from build123d import *

# Parameters (mm, degrees)
SKETCH1_R           = 95.25
SKETCH1_R_2         = 76.2
BOSS_EXTRUDE1_DEPTH = 7.874
SKETCH2_R           = 3.3655
CUT_EXTRUDE1_DEPTH  = 8.874
CIRPATTERN1_COUNT   = 8


with BuildPart() as part:
    # Sketch1 → Boss-Extrude1 (new body)
    with BuildSketch(Plane.XY):
        Circle(SKETCH1_R)
        Circle(SKETCH1_R_2, mode=Mode.SUBTRACT)
    extrude(amount=BOSS_EXTRUDE1_DEPTH)

    # Sketch2 → Cut-Extrude1 (cut, through all)
    with BuildSketch(Plane.XY.offset(7.874)):
        with Locations((0, 85.09)):
            Circle(SKETCH2_R)
    cut_extrude1 = extrude(amount=-CUT_EXTRUDE1_DEPTH, mode=Mode.SUBTRACT)

    # CirPattern1: Cut-Extrude1 ×8 about axis
    cirpattern1_axis = Axis((0, 0, 0), (0, 0, 1))
    for i in range(1, CIRPATTERN1_COUNT):
        add(cut_extrude1.rotate(cirpattern1_axis, i * 360 / CIRPATTERN1_COUNT), mode=Mode.SUBTRACT)


solid = part.part
Geometry: final body of the model. Coordinates: model frame, mm. Round coordinates to 2 decimals unless told otherwise and drop trailing zeros. Loops run counter-clockwise (first coordinate to the right, second up) from the corner with the lowest first, then second, coordinate; pieces in that order, holes last. Notation, with made-up numbers: (-2.75, 51.5) - (32.25, 51.5) arc R27 ccw to (32.25, 72.5) - close; hole circle Ø8 at (20, -10.75). An arc over 180 degrees is marked (long way). Write each question's results on one line, items separated by ' | '. Start each with the question number.
1) First-contact query: P1, Ø4, axis at x = 3.5, z = 4.5, coming from the +Y side; P2, Ø7.5, axis at x = -60.17, y = 60.17, coming from the +Z side; P3, Ø4, axis at x = -85.09, y = 0, coming from the -Z side; P4, Ø2, axis at x = -31.5, z = 4.5, coming from the -Y side. Flat tips, straight axial feed; report the tip coordinate or a pass-through.
2) Cut plane A-A on y = 0. Return loops of the section in (x, z), then the cut area to 3 significant figures.
3) Line query: probe 1 along Y at (x, z) = (0, 3.5); probe 2 along Y at (x, z) = (61, 6); probe 3 along X at (y, z) = (62.5, 2). Output: solid intervals per line, ascending. Write a range as [from, to].
4) Mould query, pull axis Y, two halves, no side actions, for faces 1 (the face through (-60.47, -46.367, 3.882)), 2 (the face through (-75.587, -57.958, 3.882)), 3 (the face through (-29, 71, 0)). Classes: released by +Y, released by -Y, zero draft, split by the parting line, or undercut.
5) Cut plane C-C on y = -85.09. Return loops of the section in (x, z).
Verdict:
1) P1: stops at y = 95.24 | P2: stops at z = 7.87 | P3: passes through | P4: stops at y = -90.23
2) outline: (-95.25, 0) - (-88.46, 0) - (-88.46, 7.87) - (-95.25, 7.87) - close; (-81.72, 0) - (-76.2, 0) - (-76.2, 7.87) - (-81.72, 7.87) - close; (76.2, 0) - (81.72, 0) - (81.72, 7.87) - (76.2, 7.87) - close; (88.46, 0) - (95.25, 0) - (95.25, 7.87) - (88.46, 7.87) - close | area: 194 mm2
3) probe 1: y = [-95.25, -88.46], [-81.72, -76.2], [76.2, 81.72], [88.46, 95.25] | probe 2: y = [-73.15, -63.43], [-56.91, -45.67], [45.67, 56.91], [63.43, 73.15] | probe 3: x = [-71.88, -62.59], [-57.74, -43.59], [43.59, 57.74], [62.59, 71.88]
4) face 1: undercut | face 2: split by the parting line | face 3: zero draft
5) outline: (-42.8, 0) - (-3.37, 0) - (-3.37, 7.87) - (-42.8, 7.87) - close; (3.37, 0) - (42.8, 0) - (42.8, 7.87) - (3.37, 7.87) - close
